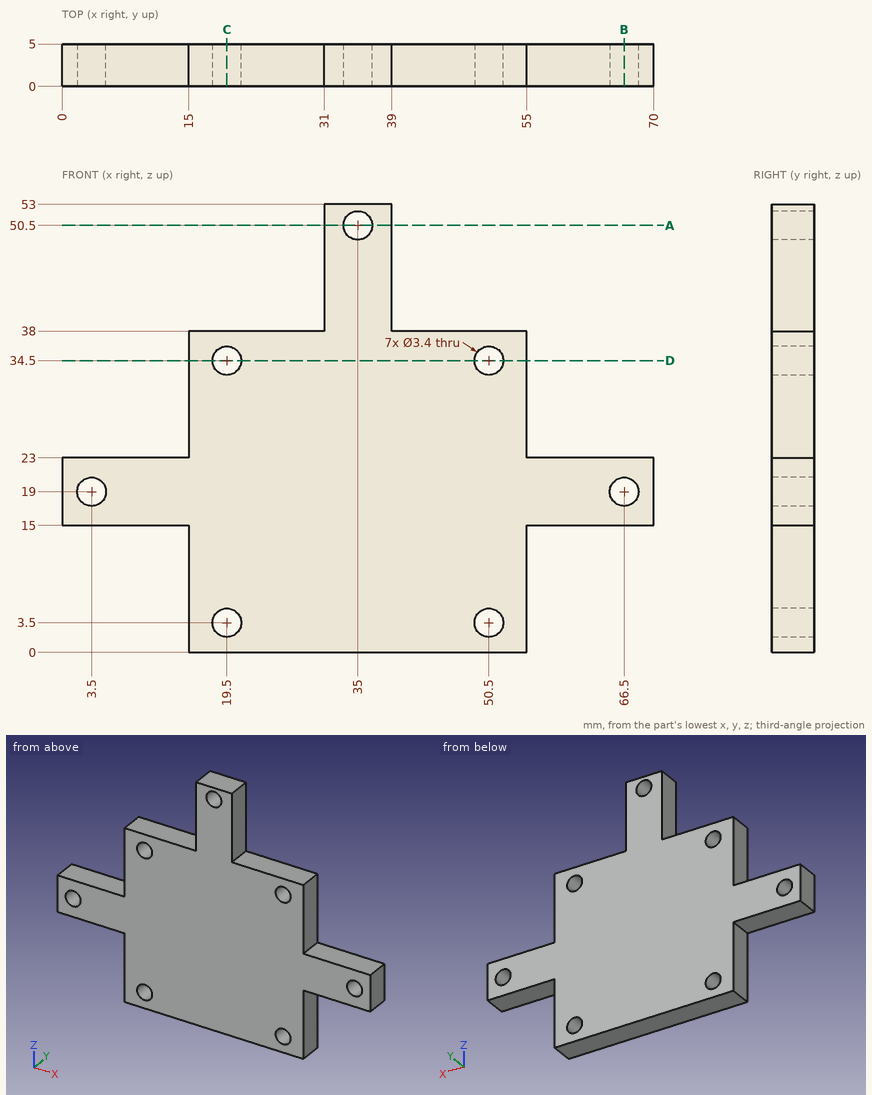
Answer from the drawing. Dimensions are ordinates in mm from the lowest x, y and z of the part. Coordinates: 2 decimals unless noted, no trailing zeros. Loops run counter-clockwise (first coordinate to the right, second up) from the corner with the lowest first, then second, coordinate; pieces in that order, holes last.
Q1. The part is cut by section A-A on z = 50.5. Write down the section's boundary in (x, y).
Q2. Consider probe 1 along X at (y, z) = (1.4, 34.5); probe 2 along X at (y, z) = (3.3, 19); probe 3 along Z at (x, y) = (35, 2.7). Determine where each line is inside the solid, lowest interval first.
Q3. The part is cut by section B-B on x = 66.5. Write down the section's boundary in (y, z).
Q4. Each of these flat-tipped pins is pushed along its axis until it touches: pin 1 Ø2.5 at (y, z) = (2.5, 9.5) entering from -X; pin 2 Ø1.5 at (x, y) = (20, 1.5) entering from +Z; pin 3 Ø3 at (y, z) = (2.5, 29.5) entering from +X. Where does it stop, or does it pass through?
Q5. The part is cut by section D-D on z = 34.5. Write down the section's boundary in (x, y), and give its area (3 significant figures).
Q6. The part is cut by section C-C on x = 19.5. Write down the section's boundary in (y, z), and give its area (3 significant figures).
Results below:
1. outline: (31, 0) - (33.3, 0) - (33.3, 5) - (31, 5) - close; (36.7, 0) - (39, 0) - (39, 5) - (36.7, 5) - close
2. probe 1: x = 15 to 17.8, 21.2 to 48.8, 52.2 to 55
2. probe 2: x = 0 to 1.8, 5.2 to 64.8, 68.2 to 70
2. probe 3: z = 0 to 48.8, 52.2 to 53
3. outline: (0, 15) - (5, 15) - (5, 17.3) - (0, 17.3) - close; (0, 20.7) - (5, 20.7) - (5, 23) - (0, 23) - close
4. pin 1: stops at x = 15
4. pin 2: stops at z = 38
4. pin 3: stops at x = 55
5. outline: (15, 0) - (17.8, 0) - (17.8, 5) - (15, 5) - close; (21.2, 0) - (48.8, 0) - (48.8, 5) - (21.2, 5) - close; (52.2, 0) - (55, 0) - (55, 5) - (52.2, 5) - close
5. area: 166 mm2
6. outline: (0, 0) - (5, 0) - (5, 1.8) - (0, 1.8) - close; (0, 5.2) - (5, 5.2) - (5, 32.8) - (0, 32.8) - close; (0, 36.2) - (5, 36.2) - (5, 38) - (0, 38) - close
6. area: 156 mm2
